Build history of the part. All positions in model axes, mm. Give positions to 0.01 mm unless a question says otherwise; leave off trailing zeros. Order: outer loops, then holes, each group sorted by start corner. A loop starts at its lowest first (then second) coordinate and runs counter-clockwise, first axis right, second up. Notation, with made-up numbers: M 17,43 L 29,43 A11 ccw 29,48 Z; hole C 52.25,-36 d2. An arc over 180 degrees is marked long. One line per item, written item: value.
from build123d import *

# Parameters (mm, degrees)
F0_W           = 304.8
F0_H           = 152.4
F1_DEPTH       = 76.2
F3_D           = 7.9375
F3_CSINK_D     = 15.875
F3_CSINK_ANGLE = 85
F4_R           = 6.35
F5_R           = 6.35


with BuildPart() as f1:
    # F0 (on Top) → F1 (new body)
    with BuildSketch(Plane.XY):
        Rectangle(F0_W, F0_H)
    extrude(amount=F1_DEPTH)

    # F3 (through all)
    with Locations(Plane.XY.offset(76.2)):
        with Locations((-127, 0), (127, 0)):
            CounterSinkHole(F3_D / 2, F3_CSINK_D / 2, counter_sink_angle=F3_CSINK_ANGLE)

    # F4
    f4_edges = [f1.edges().sort_by_distance(p)[0] for p in [
        (-152.4, 0, 76.2),
        (152.4, 0, 76.2),
    ]]
    fillet(f4_edges, radius=F4_R)

    # F5
    f5_edges = [f1.edges().sort_by_distance(p)[0] for p in [
        (0, -76.2, 76.2),
        (0, 76.2, 76.2),
    ]]
    fillet(f5_edges, radius=F5_R)


solid = f1.part
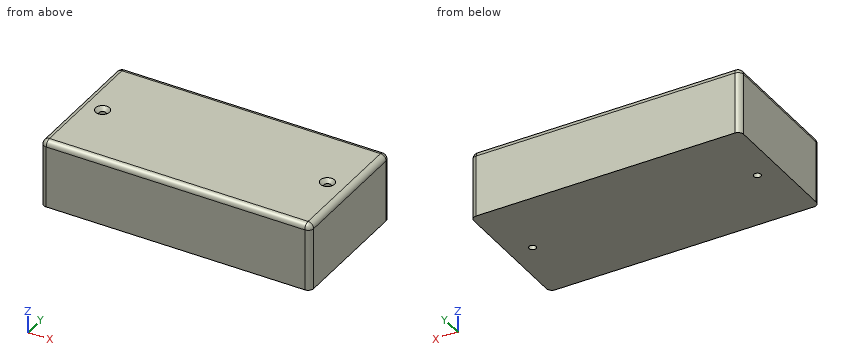
1) Drill centre lines: probe 1 along X at (y, z) = (0, 35); probe 2 along Y at (x, z) = (-127, 36); probe 3 along X at (y, z) = (34, 72.5). Where is each one in solid material? Low to high. Write a range as from..to.
Check values:
probe 1: -152.4..-130.97, -123.03..123.03, 130.97..152.4
probe 2: -76.2..-3.97, 3.97..76.2
probe 3: -151.82..151.82
2) Pin check, flat tips, straight feed: pin 1 (9 mm diameter, centred on x = 127, y = 0, fed in from +Z); pin 2 (4 mm diameter, centred on x = -109.5, y = 49.5, fed in from -Z). Stop position of each tip, or through.
Check values:
pin 1: z = 72.45
pin 2: z = 0
3) Saw through at B-B, the plane y = 0. Write the cut outline in (x, z).
Check values:
outline: M -152.4,0 L -130.97,0 L -130.97,71.87 L -134.94,76.2 L -146.05,76.2 A6.35 ccw -152.4,69.85 Z; M -123.03,0 L 123.03,0 L 123.03,71.87 L 119.06,76.2 L -119.06,76.2 L -123.03,71.87 Z; M 130.97,0 L 152.4,0 L 152.4,69.85 A6.35 ccw 146.05,76.2 L 134.94,76.2 L 130.97,71.87 Z
4) Saw through at A-A, the plane x = -127. Write the cut outline in (y, z), then the cut area to 3 significant figures.
Check values:
outline: M -76.2,0 L -3.97,0 L -3.97,71.87 L -7.94,76.2 L -69.85,76.2 A6.35 ccw -76.2,69.85 Z; M 3.97,0 L 76.2,0 L 76.2,69.85 A6.35 ccw 69.85,76.2 L 7.94,76.2 L 3.97,71.87 Z
area: 11,000 mm^2
